from build123d import *

# Parameters (mm, degrees)
BOX001_W         = 50
BOX001_H         = 50
BOX001_DEPTH     = 20
BOX002_W         = 56
BOX002_H         = 56
BOX002_DEPTH     = 23
EXTRUDE001_DEPTH = 3


with BuildPart() as cube001:
    # Box001 → Box001 (new body)
    with BuildSketch(Plane(origin=(3, 3, 3), x_dir=(1, 0, 0), z_dir=(0, 0, 1))):
        with Locations((25, 25)):
            Rectangle(BOX001_W, BOX001_H)
    extrude(amount=BOX001_DEPTH)


with BuildPart() as obj1:
    # Box002 → Box002 (new body)
    with BuildSketch(Plane.XY):
        with Locations((28, 28)):
            Rectangle(BOX002_W, BOX002_H)
    extrude(amount=BOX002_DEPTH)

    # Cut: cut Cube001
    add(cube001.part, mode=Mode.SUBTRACT)


with BuildPart() as fusion_caixa_end:
    # Sketch002 → Extrude001 (new body)
    with BuildSketch(Plane.XY):
        with BuildLine():
            Line((17.981379, 51.82386), (38.018621, 51.82386))
            Line((38.018621, 51.82386), (32.795895, 71.168476))
            ThreePointArc((32.795895, 71.168476), (28, 74.841274), (23.204105, 71.168476))
            Line((23.204105, 71.168476), (17.981379, 51.82386))
        make_face()
        with BuildLine():
            ThreePointArc((30.625023, 69.873664), (28, 72.498687), (25.374977, 69.873664))
            Line((25.374977, 69.873664), (25.374977, 61.048153))
            ThreePointArc((25.374977, 61.048153), (28, 58.42313), (30.625023, 61.048153))
            Line((30.625023, 69.873664), (30.625023, 61.048153))
        make_face(mode=Mode.SUBTRACT)
    extrude(amount=EXTRUDE001_DEPTH)

    # Fusion002: union obj1
    add(obj1.part)


solid = fusion_caixa_end.part
Model file for the job. Use its own axes, mm. A direction names the side the tool comes from. Round coordinates to 2 decimals unless told otherwise and drop trailing zeros. Order: outer loops, then holes, each group sorted by start corner. A loop starts at its lowest first (then second) coordinate and runs counter-clockwise, first axis right, second up.
(1) Band-saw the part on A-A (z = 13). List the corners of the cut face in (x, y).
(2) Band-saw the part on C-C (x = 28). List the corners of the cut face in (y, z).
(3) Drill centre lines: line 1 (X direction, y = 11.5, z = 8); line 2 (Z direction, x = 44.5, y = 38.5). Where is each one in solid material? Low to high.
(4) Band-saw the part on D-D (y = 66). List the corners of the cut face in (x, z).
(5) 3-axis set-ups, long thin cutter, end or side, ignore diameter. For faces 4 (the face through (32, 63, 3)), 5 (the face through (28.06, 72.5, 1.48)), 6 (the face through (53, 28, 13)): which of +Z, -Z, +X, -X, +Y, -Y reach the whole face in a straight line?
(6) Pin check, flat tips, straight feed: pin 1 (1 mm diameter, centred on x = 37.5, y = 60.5, fed in from -Z); pin 2 (10 mm diameter, centred on x = 22, z = 16, fed in from +Y); pin 3 (25 mm diameter, centred on x = 20.5, y = 39.5, fed in from +Z); pin 4 (1.5 mm diameter, centred on y = 66, z = 1, fed in from -X). Stop position of each tip, or through.
(7) Band-saw the part on B-B (y = 15). List the corners of the cut face in (x, z), then the cut area to 3 significant figures.
(8) Pull direction X, two halves, no side cores. Call faces 1 (the face through (28, 56, 11)), 2 (the face through (28, 3, 13)), 3 (the face through (0, 28, 11)): released by +X, released by -X, zero draft, split by the parting line, or undercut.
Verdict:
1. outline: (0, 0) - (56, 0) - (56, 56) - (0, 56) - close; hole (3, 3) - (53, 3) - (53, 53) - (3, 53) - close
2. outline: (0, 0) - (58.42, 0) - (58.42, 3) - (56, 3) - (56, 23) - (53, 23) - (53, 3) - (3, 3) - (3, 23) - (0, 23) - close; (72.5, 0) - (74.84, 0) - (74.84, 3) - (72.5, 3) - close
3. line 1: x = 0 to 3, 53 to 56
3. line 2: z = 0 to 3
4. outline: (21.81, 0) - (25.37, 0) - (25.37, 3) - (21.81, 3) - close; (30.63, 0) - (34.19, 0) - (34.19, 3) - (30.63, 3) - close
5. face 4: +Z, +X, -X, +Y
5. face 5: +Z, -Z
5. face 6: +Z
6. pin 1: passes through
6. pin 2: stops at y = 56
6. pin 3: stops at z = 3
6. pin 4: stops at x = 21.61
7. outline: (0, 0) - (56, 0) - (56, 23) - (53, 23) - (53, 3) - (3, 3) - (3, 23) - (0, 23) - close
7. area: 288 mm2
8. face 1: zero draft
8. face 2: undercut
8. face 3: released by -X
